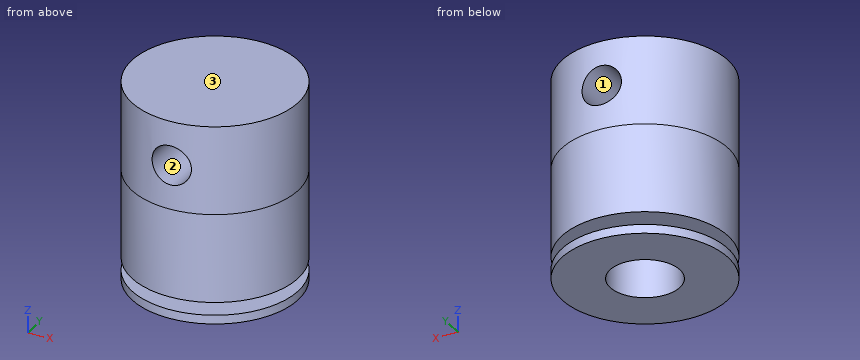
from build123d import *

# Parameters (mm, degrees)
SKETCH1_R               = 4.7625
BOSS_EXTRUDE1_DEPTH     = 5.08
SKETCH2_R               = 2.667
BOSS_EXTRUDE2_DEPTH     = 0.7366
SKETCH3_R               = 4.7625
BOSS_EXTRUDE3_DEPTH     = 5.08
CUT_EXTRUDE1_DEPTH      = 6.35
CUT_EXTRUDE1_DEPTH_BACK = 6.35
SKETCH6_R               = 1.1303
SKETCH7_R               = 3.5000057
CUT_EXTRUDE2_DEPTH      = 2.50000008
SKETCH8_R               = 1.999996
CUT_EXTRUDE3_DEPTH      = 10.0000054
SKETCH9_R               = 4.7625
CUT_EXTRUDE4_DEPTH      = 4.572
SKETCH10_R              = 1.999996
CUT_EXTRUDE5_DEPTH      = 10.0000054


with BuildPart() as part:
    # Sketch1 → Boss-Extrude1 (new body)
    with BuildSketch(Plane.XY):
        Circle(SKETCH1_R)
    extrude(amount=BOSS_EXTRUDE1_DEPTH)

    # Sketch2 → Boss-Extrude2 (add)
    with BuildSketch(Plane.XY.offset(5.08)):
        Circle(SKETCH2_R)
    extrude(amount=BOSS_EXTRUDE2_DEPTH)

    # Sketch3 → Boss-Extrude3 (add)
    with BuildSketch(Plane.XY.offset(5.8166)):
        Circle(SKETCH3_R)
    boss_extrude3 = extrude(amount=BOSS_EXTRUDE3_DEPTH)

    # Mirror3: Boss-Extrude3 across plane
    add(boss_extrude3.mirror(Plane.XY.offset(10.8966)))

    # Sketch6 → Cut-Extrude1 (cut, two sides: drawn at the far end of the back side and taken through both)
    with BuildSketch(Plane(origin=(0, 0, 0), x_dir=(1, 0, 0), z_dir=(0, 1, 0)).offset(-CUT_EXTRUDE1_DEPTH_BACK)):
        with Locations(Location((0, -13.4366, 0), (0, 0, 90))):
            Circle(SKETCH6_R)
    extrude(amount=CUT_EXTRUDE1_DEPTH + CUT_EXTRUDE1_DEPTH_BACK, mode=Mode.SUBTRACT)

    # Sketch7 → Cut-Extrude2 (cut)
    with BuildSketch(Plane(origin=(0, 0, 0), x_dir=(-1, 0, 0), z_dir=(0, 0, -1))):
        Circle(SKETCH7_R)
    extrude(amount=-CUT_EXTRUDE2_DEPTH, mode=Mode.SUBTRACT)

    # Sketch8 → Cut-Extrude3 (cut)
    with BuildSketch(Plane(origin=(0, 0, 2.50000008), x_dir=(-1, 0, 0), z_dir=(0, 0, -1))):
        Circle(SKETCH8_R)
    extrude(amount=-CUT_EXTRUDE3_DEPTH, mode=Mode.SUBTRACT)

    # Sketch9 → Cut-Extrude4 (cut)
    with BuildSketch(Plane(origin=(0, 0, 0), x_dir=(-1, 0, 0), z_dir=(0, 0, -1))):
        Circle(SKETCH9_R)
    extrude(amount=-CUT_EXTRUDE4_DEPTH, mode=Mode.SUBTRACT)

    # Sketch10 → Cut-Extrude5 (cut)
    with BuildSketch(Plane(origin=(0, 0, 4.572), x_dir=(-1, 0, 0), z_dir=(0, 0, -1))):
        Circle(SKETCH10_R)
    extrude(amount=-CUT_EXTRUDE5_DEPTH, mode=Mode.SUBTRACT)


solid = part.part
Part model, mm, in its own coordinate system. Face numbers are marked on the shaded views. Give positions to 0.01 mm unless a question says otherwise; leave off trailing zeros. Write each loop counter-clockwise with the first axis right and the second up, starting at its lowest first coordinate (ties: lowest second). Pieces come first, ordered by that corner, then holes.
1) Cut at A-A on x = 0. State how many separate pieces and enclosed holes the cut face has, then the cut area to 3 significant figures.
Resolved:
separate pieces: 3
enclosed holes: 0
area: 53.1 mm2
2) Pin check, flat tips, straight feed: pin 1 (1.2 mm diameter, centred on x = 0, y = 0.5, fed in from -Z); pin 2 (1 mm diameter, centred on y = 2, z = 6.5, fed in from -X); pin 3 (1 mm diameter, centred on y = 2.5, z = 6.5, fed in from -X); pin 4 (1.4 mm diameter, centred on x = 0, z = 13.44, fed in from +Y). Stop position of each tip, or through.
Resolved:
pin 1: stops at z = 14.57
pin 2: stops at x = -4.52
pin 3: stops at x = -4.32
pin 4: passes through
3) Two-plate mould, pull along X, no slides. Class the marked faces 1, 2 and 3: released by +X, released by -X, zero draft, split by the parting line, or undercut.
Resolved:
face 1: undercut
face 2: undercut
face 3: zero draft
4) Probe L1, parallel to Z at x = -2.75, y = -3.5; L2, parallel to Y at x = 0, z = 7; L3, parallel to Z at x = 1, y = 2.75. List the from-to ranges inside material, lowest first.
Resolved:
L1: z = 4.57 to 5.08, 5.82 to 15.98
L2: y = -4.76 to -2, 2 to 4.76
L3: z = 4.57 to 5.08, 5.82 to 12.91, 13.96 to 15.98
5) Cut at D-D on z = 14.75. Write the cut outline in (x, y) (1 decimal), then the cut area to 3 significant figures.
Resolved:
outline: circle Ø9.5 at (0, 0)
area: 71.3 mm2
6) Cut at C-C on x = 4.25. Write the cut outline in (y, z), then the cut area to 3 significant figures.
Resolved:
outline: (-2.15, 4.57) - (2.15, 4.57) - (2.15, 5.08) - (-2.15, 5.08) - close; (-2.15, 5.82) - (2.15, 5.82) - (2.15, 15.98) - (-2.15, 15.98) - close
area: 45.9 mm2
7) Cut at B-B on y = 3. Write the cut outline in (x, z).
Resolved:
outline: (-3.7, 4.57) - (3.7, 4.57) - (3.7, 5.08) - (-3.7, 5.08) - close; (-3.7, 5.82) - (3.7, 5.82) - (3.7, 15.98) - (-3.7, 15.98) - close; hole circle Ø2.26 at (0, 13.44)
